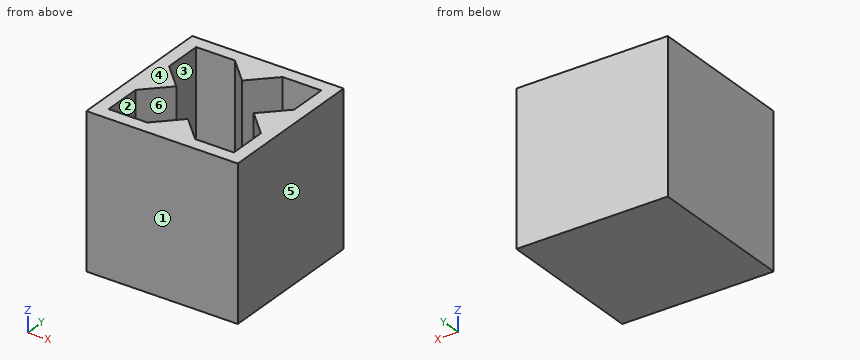
```python
from build123d import *

# Parameters (mm, degrees)
F0_W     = 25.4
F0_H     = 25.4
F1_DEPTH = 25.4
F3_DEPTH = 20


with BuildPart() as f1:
    # F0 (on Top) → F1 (new body)
    with BuildSketch(Plane.XY):
        with Locations((12.7, 12.7)):
            Rectangle(F0_W, F0_H)
    extrude(amount=F1_DEPTH)

    # F2 (on face) → F3 (cut)
    with BuildSketch(Plane.XY.offset(25.4)):
        Polygon((19.2, 12.7), (12.7, 12.7), (12.7, 6.2), (16.7, 2.2), (23.2, 2.2), (23.2, 8.7), align=None)
        Polygon((12.7, 19.2), (12.7, 12.7), (19.2, 12.7), (23.2, 16.7), (23.2, 23.2), (16.7, 23.2), align=None)
        Polygon((12.7, 12.7), (6.2, 12.7), (2.2, 8.7), (2.2, 2.2), (8.7, 2.2), (12.7, 6.2), align=None)
        Polygon((2.2, 16.7), (6.2, 12.7), (12.7, 12.7), (12.7, 19.2), (8.7, 23.2), (2.2, 23.2), align=None)
    extrude(amount=-F3_DEPTH, mode=Mode.SUBTRACT)


solid = f1.part
```
Read the model definition and answer for the solid it produces. Units are mm, in the model's axes. Face numbers are marked on the shaded views. A direction names the side the tool comes from. Coordinates: 2 decimals unless noted, no trailing zeros. Write each loop counter-clockwise with the first axis right and the second up, starting at its lowest first coordinate (ties: lowest second). Pieces come first, ordered by that corner, then holes. Notation, with made-up numbers: (-0.5, 30) -> (26.5, 30) arc R28 ccw to (26.5, 62) -> close; hole circle Ø7 at (7.5, 61.25). An arc over 180 degrees is marked (long way). Answer as a JSON object with one key per item and string values.
Q1. The part is cut by section A-A on x = 15.5. Give the vertices of the cut face in (y, z), then the cut area to 3 significant figures.
The answers:
{"outline": "(0, 0) -> (25.4, 0) -> (25.4, 25.4) -> (22, 25.4) -> (22, 5.4) -> (3.4, 5.4) -> (3.4, 25.4) -> (0, 25.4) -> close", "area": "273 mm2"}
Q2. Determine the mould class of the marked faces 3, 4, 5 and 6 for opening direction X: pulls with the +X half, pulls with the -X half, needs draft (parallel to the pull), parting line crosses it, or undercut.
The answers:
{"face 3": "undercut", "face 4": "needs draft", "face 5": "pulls with the +X half", "face 6": "undercut"}
Q3. The part is cut by section D-D on x = 20. Give the vertices of the cut face in (y, z), then the cut area to 3 significant figures.
The answers:
{"outline": "(0, 0) -> (25.4, 0) -> (25.4, 25.4) -> (23.2, 25.4) -> (23.2, 5.4) -> (13.5, 5.4) -> (13.5, 25.4) -> (11.9, 25.4) -> (11.9, 5.4) -> (2.2, 5.4) -> (2.2, 25.4) -> (0, 25.4) -> close", "area": "257 mm2"}
Q4. The part is cut by section B-B on z = 7.5. Give the vertices of the cut face in (x, y).
The answers:
{"outline": "(0, 0) -> (25.4, 0) -> (25.4, 25.4) -> (0, 25.4) -> close; hole (2.2, 2.2) -> (8.7, 2.2) -> (12.7, 6.2) -> (16.7, 2.2) -> (23.2, 2.2) -> (23.2, 8.7) -> (19.2, 12.7) -> (23.2, 16.7) -> (23.2, 23.2) -> (16.7, 23.2) -> (12.7, 19.2) -> (8.7, 23.2) -> (2.2, 23.2) -> (2.2, 16.7) -> (6.2, 12.7) -> (2.2, 8.7) -> close"}
Q5. A tool of negligible diameter and unlimited length cuts with its end or side. For the marked faces 1 and 2, from which of +Z, -Z, +X, -X, +Y, -Y can it reach the whole face along a straight path? Write none if from no direction.
The answers:
{"face 1": "+Z, -Z, +X, -X, -Y", "face 2": "+Z"}
Q6. Consider line 1 (Y direction, x = 8.5, z = 23.5); line 2 (Y direction, x = 6, z = 6.5). Determine where each line is inside the solid, lowest interval first. Write a range as [from, to].
The answers:
{"line 1": "y = [0, 2.2], [23.2, 25.4]", "line 2": "y = [0, 2.2], [12.5, 12.9], [23.2, 25.4]"}
Q7. The part is cut by section C-C on y = 11. Give the vertices of the cut face in (x, z).
The answers:
{"outline": "(0, 0) -> (25.4, 0) -> (25.4, 25.4) -> (20.9, 25.4) -> (20.9, 5.4) -> (4.5, 5.4) -> (4.5, 25.4) -> (0, 25.4) -> close"}
